Design review of the part built by this model. Coordinates are the model's own, in mm. Give positions to 0.01 mm unless a question says otherwise; leave off trailing zeros. Write each loop counter-clockwise with the first axis right and the second up, starting at its lowest first coordinate (ties: lowest second). Pieces come first, ordered by that corner, then holes. Notation, with made-up numbers: M -9.5,1.5 L 8.5,1.5 A31 ccw 8.5,30.5 Z; hole C 6,20.25 d3. An arc over 180 degrees is marked long. One line per item, written item: value. Start each with the question number.
```python
from build123d import *

# Parameters (mm, degrees)
F0_R     = 3
F1_DEPTH = 0.25


with BuildPart() as f1:
    # F0 (on Top) → F1 (new body)
    with BuildSketch(Plane.XY):
        with BuildLine():
            ThreePointArc((0, 4), (1.171573, 1.171573), (4, 0))
            Line((4, 0), (76, 0))
            ThreePointArc((76, 0), (78.828427, 1.171573), (80, 4))
            Line((80, 4), (80, 76))
            ThreePointArc((80, 76), (78.828427, 78.828427), (76, 80))
            Line((76, 80), (4, 80))
            ThreePointArc((4, 80), (1.171573, 78.828427), (0, 76))
            Line((0, 76), (0, 4))
        make_face()
        with Locations((6.5, 6.5)):
            Circle(F0_R, mode=Mode.SUBTRACT)
        with Locations((73.5, 6.5)):
            Circle(F0_R, mode=Mode.SUBTRACT)
        with BuildLine():
            ThreePointArc((15, 62), (15.87868, 64.12132), (18, 65))
            Line((18, 65), (62, 65))
            ThreePointArc((62, 65), (64.12132, 64.12132), (65, 62))
            Line((65, 62), (65, 18))
            ThreePointArc((65, 18), (64.12132, 15.87868), (62, 15))
            Line((62, 15), (18, 15))
            ThreePointArc((18, 15), (15.87868, 15.87868), (15, 18))
            Line((15, 18), (15, 62))
        make_face(mode=Mode.SUBTRACT)
        with Locations((6.5, 73.5)):
            Circle(F0_R, mode=Mode.SUBTRACT)
        with Locations((73.5, 73.5)):
            Circle(F0_R, mode=Mode.SUBTRACT)
    extrude(amount=F1_DEPTH)


solid = f1.part
```
Q1. Wall thickness on line 1 (Y direction, x = 73.5, z = 0.1); line 2 (Y direction, x = 20.5, z = 0.15): over which ranges is each line inside the solid? List them lowest first. Write a range as from..to.
Q2. Take a section at A-A, the plane y = 6.5. Give the boundary of the cut face in (x, z), then the cut area to 3 significant figures.
Q3. Take a section at D-D, the plane z = 0.1. Give the boundary of the cut face in (x, y), then the cut area to 3 significant figures.
Q4. Take a section at C-C, the plane y = 43. Give the boundary of the cut face in (x, z), then the cut area to 3 significant figures.
Results list:
1. line 1: y = 0..3.5, 9.5..70.5, 76.5..80
1. line 2: y = 0..15, 65..80
2. outline: M 0,0 L 3.5,0 L 3.5,0.25 L 0,0.25 Z; M 9.5,0 L 70.5,0 L 70.5,0.25 L 9.5,0.25 Z; M 76.5,0 L 80,0 L 80,0.25 L 76.5,0.25 Z
2. area: 17.0 mm^2
3. outline: M 0,4 A4 ccw 4,0 L 76,0 A4 ccw 80,4 L 80,76 A4 ccw 76,80 L 4,80 A4 ccw 0,76 Z; hole C 6.5,6.5 d6; hole C 6.5,73.5 d6; hole M 15,18 A3 ccw 18,15 L 62,15 A3 ccw 65,18 L 65,62 A3 ccw 62,65 L 18,65 A3 ccw 15,62 Z; hole C 73.5,6.5 d6; hole C 73.5,73.5 d6
3. area: 3,780 mm^2
4. outline: M 0,0 L 15,0 L 15,0.25 L 0,0.25 Z; M 65,0 L 80,0 L 80,0.25 L 65,0.25 Z
4. area: 7.50 mm^2
